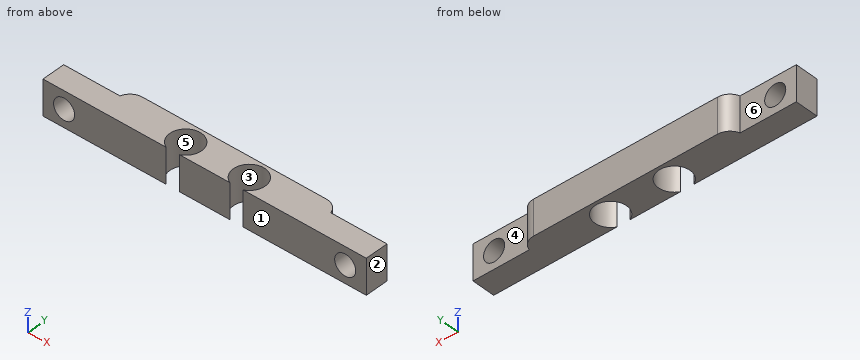
```python
from build123d import *

# Parameters (mm, degrees)
BOSS_EXTRUDE1_DEPTH     = 5
FILLET1_R               = 2
CUT_EXTRUDE1_DEPTH      = 34.538204198
CUT_EXTRUDE1_DEPTH_BACK = 34.538204198
SKETCH2_R               = 1.5
CUT_EXTRUDE2_DEPTH      = 34.709745494
CUT_EXTRUDE2_DEPTH_BACK = 34.709745494
SKETCH3_R               = 2.25


with BuildPart() as part:
    # Sketch1 → Boss-Extrude1 (new body)
    with BuildSketch(Plane.XY):
        Polygon((-5, 4.727255151), (-5, 3.288029927), (-13, 3.288029927), (-13, 0), (33, 0), (33, 3.288029927), (25, 3.288029927), (25, 4.727255151), align=None)
    extrude(amount=-BOSS_EXTRUDE1_DEPTH)

    # Fillet1
    # the kernel refuses this fillet: 2 mm, written as the material it takes off along each edge
    with BuildSketch(Plane(origin=(-5, 4.727255151, 4.799434635), x_dir=(0, -1, 0), z_dir=(0, 0, -1))) as fillet1_piece_1:
        with BuildLine():
            CenterArc((2, -1.919773854), FILLET1_R, 106.283326604, 73.716673396)
            Line((0, -1.919773854), (-0.04, -1.919773854))
            Line((-0.04, -1.919773854), (-0.04, 0))
            Line((-0.04, 0), (0, 0.04))
            ThreePointArc((0, 0.04), (0.719612612, 0.04), (1.428009728, 0.038395477))
            Line((1.428009728, 0.038395477), (1.439225223, 0))
        make_face()
    extrude(amount=14.598869269, mode=Mode.SUBTRACT)
    with BuildSketch(Plane(origin=(25, 4.727255151, 4.799434635), x_dir=(0, -1, 0), z_dir=(0, 0, -1))) as fillet1_piece_2:
        with BuildLine():
            CenterArc((2, 1.919773854), FILLET1_R, 180, 73.716673396)
            Line((0, 1.919773854), (-0.04, 1.919773854))
            Line((-0.04, 1.919773854), (-0.04, 0))
            Line((-0.04, 0), (0, -0.04))
            ThreePointArc((0, -0.04), (0.719612612, -0.04), (1.428009728, -0.038395477))
            Line((1.428009728, -0.038395477), (1.439225223, 0))
        make_face()
    extrude(amount=14.598869269, mode=Mode.SUBTRACT)

    # Sketch2 → Cut-Extrude1 (cut, two sides: drawn at the far end of the back side and taken through both)
    with BuildSketch(Plane(origin=(0, 3.288029927, 0), x_dir=(1, 0, 0), z_dir=(0, 1, 0)).offset(-CUT_EXTRUDE1_DEPTH_BACK)):
        with Locations(Location((-10, 2.5, 0), (0, 0, 180))):
            Circle(SKETCH2_R)
        with Locations(Location((30, 2.5, 0), (0, 0, 180))):
            Circle(SKETCH2_R)
    extrude(amount=CUT_EXTRUDE1_DEPTH + CUT_EXTRUDE1_DEPTH_BACK, mode=Mode.SUBTRACT)

    # Sketch3 → Cut-Extrude2 (cut, two sides: drawn at the far end of the back side and taken through both)
    with BuildSketch(Plane.XY.offset(-CUT_EXTRUDE2_DEPTH_BACK)):
        with Locations((14.527125966, 2.045207178)):
            Circle(SKETCH3_R)
        with Locations((5.472874034, 2.045207178)):
            Circle(SKETCH3_R)
    extrude(amount=CUT_EXTRUDE2_DEPTH + CUT_EXTRUDE2_DEPTH_BACK, mode=Mode.SUBTRACT)


solid = part.part
```
For this review, take the finished solid that the model builds, in its own axes (mm). Face numbers are marked on the shaded views. A direction names the side the tool comes from. Give positions to 0.01 mm unless a question says otherwise; leave off trailing zeros. Write each loop counter-clockwise with the first axis right and the second up, starting at its lowest first coordinate (ties: lowest second). Pieces come first, ordered by that corner, then holes.
Item 1: Wall thickness on probe 1 along X at (y, z) = (2.25, -2.5); probe 2 along Z at (x, y) = (30, 1.55); probe 3 along X at (y, z) = (2.15, -1.35): over which ranges is each line inside the solid? List them lowest first.
Item 2: Take a section at A-A (z = -2.5). Give the boundary of the cut face in (x, y).
Item 3: Machinability: for the marked faces 4, 5 and 6, which of the approach directions +Z, -Z, +X, -X, +Y, -Y give a long, thin tool a straight path to every point of the face, cutting with its end or side? Answer none if there is none.
Item 4: Take a section at B-B (x = 30). Give the boundary of the cut face in (y, z), and give its area (3 significant figures).
Item 5: The part is to be moulded in two halves that separate along X. For the marked faces 1, 2 and 3, say which applies: +X half, -X half, draft (parallel to the pull), parting line (faces both ways), or undercut.
Item 6: Insertion check: P1, Ø2.5, axis at x = 30, z = -2.5, coming from the +Y side; P2, Ø1.5, axis at x = -7, z = -3.5, coming from the +Y side. Each pin has a flat end and moves straight along its axis. Give the tip position at first contact, or say it passes through.
Item 7: Take a section at D-D (x = -8). Give the boundary of the cut face in (y, z).
Item 8: Take a section at C-C (y = 0.95). Give the boundary of the cut face in (x, z), and give its area (3 significant figures).
Established:
1. probe 1: x = -13 to -11.5, -8.5 to 3.23, 7.71 to 12.29, 16.77 to 28.5, 31.5 to 33
1. probe 2: z = -5 to -4, -1 to 0
1. probe 3: x = -13 to -10.96, -9.04 to 3.23, 7.72 to 12.28, 16.77 to 29.04, 30.96 to 33
2. outline: (-13, 0) - (-11.5, 0) - (-11.5, 3.29) - (-13, 3.29) - close; (-8.5, 0) - (4.53, 0) arc R2.25 cw (long way) to (6.41, 0) - (13.59, 0) arc R2.25 cw (long way) to (15.47, 0) - (28.5, 0) - (28.5, 3.29) - (25, 3.29) arc R2 ccw to (23.08, 4.73) - (-3.08, 4.73) arc R2 ccw to (-5, 3.29) - (-8.5, 3.29) - close; (31.5, 0) - (33, 0) - (33, 3.29) - (31.5, 3.29) - close
3. face 4: +Z, -Z, +X, +Y
3. face 5: +Z, -Z
3. face 6: +Z, -Z, -X, +Y
4. outline: (0, -5) - (3.29, -5) - (3.29, -4) - (0, -4) - close; (0, -1) - (3.29, -1) - (3.29, 0) - (0, 0) - close
4. area: 6.58 mm2
5. face 1: draft
5. face 2: +X half
5. face 3: undercut
6. P1: passes through
6. P2: stops at y = 3.29
7. outline: (0, -5) - (3.29, -5) - (3.29, 0) - (0, 0) - close
8. outline: (-13, -5) - (3.51, -5) - (3.51, 0) - (-13, 0) - close; (7.44, -5) - (12.56, -5) - (12.56, 0) - (7.44, 0) - close; (16.49, -5) - (33, -5) - (33, 0) - (16.49, 0) - close; hole circle Ø3 at (-10, -2.5); hole circle Ø3 at (30, -2.5)
8. area: 177 mm2
